from build123d import *
from build123d.topology import SkipClean

# Parameters (mm, degrees)
SKETCH_1_W               = 20
SKETCH_1_H               = 40
EXTRUDE_1_DEPTH          = 40
SKETCH_2_R               = 1
CUT_EXTRUDE_3_DEPTH      = 40
EXTRUDE_2_DEPTH          = 5
EXTRUDE_2_DEPTH_BACK     = 45
SKETCH_4_R               = 1.5
CHAMFER_1_SIZE           = 2
FILLET_1_R               = 1
SKETCH_5_R               = 3
EXTRUDE_3_DEPTH          = 50
EXTRUDE_4_DEPTH          = 1.5
EXTRUDE_4_DEPTH_BACK     = 53
SKETCH_7_R               = 3
SKETCH_12_W              = 1.5
SKETCH_12_H              = 6.856105301
CUT_EXTRUDE_6_DEPTH      = 25.5
EXTRUDE_START            = 6.5
SKETCH_9_R               = 3
EXTRUDE_7_DEPTH          = 6.5
EXTRUDE_9_DEPTH          = 2
EXTRUDE_9_DEPTH_BACK     = 42
SKETCH_13_R              = 1
SKETCH_13_W              = 2
SKETCH_13_H              = 21.033708108
CUT_EXTRUDE_8_DEPTH      = 42
CUT_EXTRUDE_8_DEPTH_BACK = 42
SKETCH_15_R              = 1.548049479
SKETCH_15_R_2            = 1.02
CUT_EXTRUDE_9_DEPTH      = 42


with BuildPart() as part:
    # Sketch 1 → Extrude 1 (new body)
    with BuildSketch(Plane(origin=(0, 0, 0), x_dir=(0, 0, -1), z_dir=(1, 0, 0))):
        with Locations((-16.51810585, 9.247910864)):
            Rectangle(SKETCH_1_W, SKETCH_1_H)
    extrude(amount=EXTRUDE_1_DEPTH)

    # Sketch 2 → Cut-Extrude 3 (cut)
    with BuildSketch(Plane.ZY):
        with Locations((9.01810585, 26.201539891)):
            Circle(SKETCH_2_R)
        with Locations((9.01810585, 11.201539891)):
            Circle(SKETCH_2_R)
        with Locations((24.01810585, 11.201539891)):
            Circle(SKETCH_2_R)
        with Locations(Location((24.01810585, 26.201539891, 0), (0, 0, 180))):
            Circle(SKETCH_2_R)
    extrude(amount=-CUT_EXTRUDE_3_DEPTH, mode=Mode.SUBTRACT)

    # Sketch 4 → Extrude 2 (add, two sides: drawn at the far end of the back side and taken through both)
    with BuildSketch(Plane.ZY.offset(-EXTRUDE_2_DEPTH_BACK)):
        with Locations((16.51810585, -0.752089136)):
            Circle(SKETCH_4_R)
    extrude(amount=EXTRUDE_2_DEPTH + EXTRUDE_2_DEPTH_BACK)

    # Chamfer 1
    chamfer_1_edges = [part.edges().sort_by_distance(p)[0] for p in [
        (20, -10.752089136, 6.51810585),
        (20, -10.752089136, 26.51810585),
        (20, 29.247910864, 26.51810585),
        (20, 29.247910864, 6.51810585),
    ]]
    chamfer(chamfer_1_edges, length=CHAMFER_1_SIZE)

    # Fillet 1
    fillet_1_edges = [part.edges().sort_by_distance(p)[0] for p in [
        (0, 9.247910864, 26.51810585),
        (40, 9.247910864, 26.51810585),
        (0, 9.247910864, 6.51810585),
        (0, -10.752089136, 16.51810585),
        (0, 29.247910864, 16.51810585),
        (0, -9.752089136, 25.51810585),
        (0, -9.752089136, 7.51810585),
        (0, 28.247910864, 7.51810585),
        (0, 28.247910864, 25.51810585),
        (40, 29.247910864, 16.51810585),
        (40, 9.247910864, 6.51810585),
        (40, -10.752089136, 16.51810585),
        (40, -9.752089136, 25.51810585),
        (40, -9.752089136, 7.51810585),
        (40, 28.247910864, 7.51810585),
        (40, 28.247910864, 25.51810585),
    ]]
    fillet(fillet_1_edges, radius=FILLET_1_R)

    # Sketch 5 → Extrude 3 (add)
    with BuildSketch(Plane.ZY.offset(5)):
        with Locations((16.51810585, -0.752089136)):
            Circle(SKETCH_5_R)
    extrude(amount=-EXTRUDE_3_DEPTH)

    # Sketch 7 → Extrude 4 (add, two sides: drawn at the far end of the back side and taken through both)
    with BuildSketch(Plane.ZY.offset(5).offset(-EXTRUDE_4_DEPTH_BACK)):
        with Locations((16.51810585, -0.752089136)):
            Circle(SKETCH_7_R)
    extrude(amount=EXTRUDE_4_DEPTH + EXTRUDE_4_DEPTH_BACK)

    # Sketch 12 → Cut-Extrude 6 (cut)
    with BuildSketch(Plane.XY):
        with Locations((47.25, -0.324036486)):
            Rectangle(SKETCH_12_W, SKETCH_12_H)
    extrude(amount=CUT_EXTRUDE_6_DEPTH, mode=Mode.SUBTRACT)

    # Sketch 9 → Extrude 7 (add)
    with BuildSketch(Plane.ZY.offset(EXTRUDE_START)):
        with Locations((16.51810585, -0.752089136)):
            Circle(SKETCH_9_R)
    extrude(amount=-EXTRUDE_7_DEPTH)

    # Sketch 13 → Extrude 9 (add, two sides: drawn at the far end of the back side and taken through both)
    # profile 1 of 5: a face of its own
    with SkipClean():  # the faces are left unmerged after this step: merging them gives an invalid solid
        with BuildSketch(Plane.ZY.offset(-EXTRUDE_9_DEPTH_BACK)):
            Polygon((7.51810585, 8.743176741), (25.51810585, 8.743176741), (25.51810585, 26.833697301), (24.103892287, 28.247910864), (8.932319412, 28.247910864), (7.51810585, 26.833697301), align=None)
            with Locations((9.01810585, 11.201539891)):
                Circle(SKETCH_13_R, mode=Mode.SUBTRACT)
            with Locations((24.01810585, 11.201539891)):
                Circle(SKETCH_13_R, mode=Mode.SUBTRACT)
            with Locations((9.01810585, 26.201539891)):
                Circle(SKETCH_13_R, mode=Mode.SUBTRACT)
            with Locations((24.01810585, 26.201539891)):
                Circle(SKETCH_13_R, mode=Mode.SUBTRACT)
        # profile 2 of 5: a face of its own
        with BuildSketch(Plane.ZY.offset(-EXTRUDE_9_DEPTH_BACK)):
            with Locations((5.51810585, 19.260030795)):
                Rectangle(SKETCH_13_W, SKETCH_13_H)
        # profile 3 of 5: a face of its own
        with BuildSketch(Plane.ZY.offset(-EXTRUDE_9_DEPTH_BACK)):
            Polygon((25.51810585, 8.743176741), (26.51810585, 8.743176741), (26.51810585, 29.776884849), (6.51810585, 29.776884849), (6.51810585, 8.743176741), (7.51810585, 8.743176741), (7.51810585, 26.833697301), (8.932319412, 28.247910864), (24.103892287, 28.247910864), (25.51810585, 26.833697301), align=None)
        # profile 4 of 5: a face of its own
        with BuildSketch(Plane.ZY.offset(-EXTRUDE_9_DEPTH_BACK)):
            Polygon((26.51810585, 29.776884849), (28.51810585, 29.776884849), (28.51810585, 31.554442305), (4.51810585, 31.554442305), (4.51810585, 29.776884849), (6.51810585, 29.776884849), align=None)
        # profile 5 of 5: a face of its own
        with BuildSketch(Plane.ZY.offset(-EXTRUDE_9_DEPTH_BACK)):
            Polygon((28.350606437, 8.743176741), (26.51810585, 8.743176741), (26.51810585, 29.776884849), (28.51810585, 29.776884849), align=None)
        extrude(amount=EXTRUDE_9_DEPTH + EXTRUDE_9_DEPTH_BACK)

    # Sketch 14 → Cut-Extrude 8 (cut, two sides: drawn at the far end of the back side and taken through both)
    with BuildSketch(Plane(origin=(0, 0, 6.51810585), x_dir=(-1, 0, 0), z_dir=(0, 0, -1)).offset(-CUT_EXTRUDE_8_DEPTH_BACK)):
        Polygon((-40, 2.426770895), (-40, 30.001767149), (0, 30.001767149), (0, 7.074046983), (16.825190811, 7.428599357), (20.42980661, -19.990117542), (-71.103797865, -17.153698552), (-61.176331402, 0), (-52.017061748, 5.892205738), align=None)
    extrude(amount=CUT_EXTRUDE_8_DEPTH + CUT_EXTRUDE_8_DEPTH_BACK, mode=Mode.SUBTRACT)

    # Sketch 15 → Cut-Extrude 9 (cut)
    with BuildSketch(Plane.XZ.offset(-30.001767149)):
        with Locations(Location((20, 16.413361069, 0), (0, 0, 270))):
            Circle(SKETCH_15_R)
        with Locations(Location((20, 23.413361069, 0), (0, 0, 270))):
            Circle(SKETCH_15_R_2)
        with Locations(Location((15.050252532, 21.363108537, 0), (0, 0, 270))):
            Circle(SKETCH_15_R_2)
        with Locations(Location((13, 16.413361069, 0), (0, 0, 270))):
            Circle(SKETCH_15_R_2)
        with Locations(Location((15.050252532, 11.4636136, 0), (0, 0, 270))):
            Circle(SKETCH_15_R_2)
        with Locations(Location((20, 9.413361069, 0), (0, 0, 270))):
            Circle(SKETCH_15_R_2)
        with Locations(Location((24.949747468, 11.4636136, 0), (0, 0, 270))):
            Circle(SKETCH_15_R_2)
        with Locations(Location((27, 16.413361069, 0), (0, 0, 270))):
            Circle(SKETCH_15_R_2)
        with Locations(Location((24.949747468, 21.363108537, 0), (0, 0, 270))):
            Circle(SKETCH_15_R_2)
    extrude(amount=-CUT_EXTRUDE_9_DEPTH, mode=Mode.SUBTRACT)


solid = part.part
Could you check a few things on this model? Use its own coordinates, in mm. A direction names the side the tool comes from. Give positions to 0.01 mm unless a question says otherwise; leave off trailing zeros. Write each loop counter-clockwise with the first axis right and the second up, starting at its lowest first coordinate (ties: lowest second). Pieces come first, ordered by that corner, then holes. Notation, with made-up numbers: (72, 84.5) -> (125, 84.5) arc R11 cw to (125, 100.5) -> close; hole circle Ø11 at (56, -8.75). An arc over 180 degrees is marked (long way). Answer as CSV lines item,"result". Start each with the question number.
(1) If we section it at D-D, the plane z = 6.75: Write out the boundary of the cut face in (x, y).
(2) I'm going to push flat-ended pins straight in: pin 1 Ø1.6 at (y, z) = (26.2, 24.02) entering from -X; pin 2 Ø4 at (x, z) = (20, 16.41) entering from -Y; pin 3 Ø2.5 at (x, z) = (24.95, 21.36) entering from +Y. Where does each tip first touch, or does it pass through?
(3) If we section it at B-B, the plane y = 22.25: Write out the boundary of the cut face in (x, z).
(4) If we section it at C-C, the plane x = 13: Write out the boundary of the cut face in (y, z).
(5) If we mould it in two halves opening along X, with no side actions, what happens to faces 3 (the face through (20.1, 30.3, 4.518)), 4 (the face through (-2, 20, 16)), 5 (the face through (14.145, 30.767, 10.993)), 6 (the face through (42, 20, 16))? For each: +X half, -X half, draft (parallel to the pull), parting line (faces both ways), or undercut.
(6) Please list where these lines run through material, in increasing order: line 1 (X direction, y = 12.75, z = 6.5); line 2 (Y direction, x = 37, z = 7).
(7) Which directions (+Z, -Z, +X, -X, +Y, -Y) give clear straight access to the entire face, cutting with the end or side of a thin tool? Please do faces 1 (the face through (12.095, 30.767, 15.943)), 2 (the face through (20, 30.002, 19)).
(8) If we section it at A-A, the plane x = 20: Write out the boundary of the cut face in (y, z), and give its area (3 significant figures).
Answer list:
1,outline,"(-2, 8.74) -> (0, 8.74) -> (0, 30) -> (40, 30) -> (40, 8.74) -> (42, 8.74) -> (42, 31.55) -> (-2, 31.55) -> close"
2,pin 1,"through"
2,pin 2,"y = 30"
2,pin 3,"y = 31.55"
3,outline,"(-2, 4.52) -> (0, 4.52) -> (0, 28.46) -> (-2, 28.46) -> close; (40, 4.52) -> (42, 4.52) -> (42, 28.46) -> (40, 28.46) -> close"
4,outline,"(30, 4.52) -> (31.55, 4.52) -> (31.55, 15.39) -> (30, 15.39) -> close; (30, 17.43) -> (31.55, 17.43) -> (31.55, 28.52) -> (30, 28.52) -> close"
5,face 3,"draft"
5,face 4,"-X half"
5,face 5,"undercut"
5,face 6,"+X half"
6,line 1,"-2 to 0, 40 to 42"
6,line 2,"30 to 31.55"
7,face 1,"+Y, -Y"
7,face 2,"+Z, -Z, -Y"
8,outline,"(30, 4.52) -> (31.55, 4.52) -> (31.55, 8.39) -> (30, 8.39) -> close; (30, 10.43) -> (31.55, 10.43) -> (31.55, 14.87) -> (30, 14.87) -> close; (30, 17.96) -> (31.55, 17.96) -> (31.55, 22.39) -> (30, 22.39) -> close; (30, 24.43) -> (31.55, 24.43) -> (31.55, 28.52) -> (30, 28.52) -> close"
8,area,"26.1 mm^2"
